For this review, take the finished solid that the model builds, in its own axes (mm). A direction names the side the tool comes from. Coordinates: 2 decimals unless noted, no trailing zeros. Write each loop counter-clockwise with the first axis right and the second up, starting at its lowest first coordinate (ties: lowest second). Pieces come first, ordered by that corner, then holes. Notation, with made-up numbers: (35, 78.5) - (85, 78.5) arc R17 cw to (85, 93.5) - close; hole circle Ø4 at (33, 72). An arc over 180 degrees is marked (long way). Write each question's results on one line, items separated by ' | '.
from build123d import *

# Parameters (mm, degrees)
SKETCH_1_W          = 104
SKETCH_1_H          = 130
EXTRUDE_1_DEPTH     = 70
SHELL_1_T           = -2
SKETCH_4_W          = 21
SKETCH_4_H          = 65
CUT_EXTRUDE_1_DEPTH = 70
SKETCH_6_W          = 16
SKETCH_6_H          = 60
CUT_EXTRUDE_2_DEPTH = 70
SKETCH_13_W         = 3
SKETCH_13_H         = 45
EXTRUDE_5_DEPTH     = 70
FILLET_2_R          = 3


with BuildPart() as part:
    # 草圖1 → 填料-伸長1 (new body)
    with BuildSketch(Plane.XY):
        Rectangle(SKETCH_1_W, SKETCH_1_H)
    extrude(amount=EXTRUDE_1_DEPTH)

    # 薄殼1
    shell_1_openings = [part.faces().sort_by_distance(p)[0] for p in [
        (0, 0, 70),
    ]]
    offset(amount=SHELL_1_T, openings=shell_1_openings, kind=Kind.INTERSECTION)

    # 草圖4 → 除料-伸長1 (cut)
    with BuildSketch(Plane.ZY.offset(52)):
        with Locations((22.5, -28.5)):
            Rectangle(SKETCH_4_W, SKETCH_4_H)
    extrude(amount=-CUT_EXTRUDE_1_DEPTH, mode=Mode.SUBTRACT)

    # 草圖6 → 除料-伸長2 (cut)
    with BuildSketch(Plane(origin=(52, 0, 0), x_dir=(0, 0, -1), z_dir=(1, 0, 0))):
        with Locations((-16.5, 31)):
            Rectangle(SKETCH_6_W, SKETCH_6_H)
    extrude(amount=-CUT_EXTRUDE_2_DEPTH, mode=Mode.SUBTRACT)

    # 草圖13 → 填料-伸長5 (add)
    with BuildSketch(Plane(origin=(52, 0, 0), x_dir=(0, 0, -1), z_dir=(1, 0, 0))):
        with Locations((-31.5, -42.5)):
            Rectangle(SKETCH_13_W, SKETCH_13_H)
    extrude(amount=-EXTRUDE_5_DEPTH)

    # 圓角2
    fillet_2_edges = [part.edges().sort_by_distance(p)[0] for p in [
        (52, -65, 35),
        (-52, -65, 35),
        (-52, 65, 35),
        (52, 65, 35),
    ]]
    fillet(fillet_2_edges, radius=FILLET_2_R)


solid = part.part
Q1. Take a section at C-C on z = 48. State the section outline as (x, y) points.
Results found:
outline: (-52, -62) arc R3 ccw to (-49, -65) - (49, -65) arc R3 ccw to (52, -62) - (52, 62) arc R3 ccw to (49, 65) - (-49, 65) arc R3 ccw to (-52, 62) - close; hole (-50, -63) - (50, -63) - (50, 63) - (-50, 63) - close
Q2. Take a section at A-A on y = -6. State the section outline as (x, z) points.
Results found:
outline: (-52, 0) - (52, 0) - (52, 70) - (50, 70) - (50, 2) - (-50, 2) - (-50, 12) - (-52, 12) - close; (-52, 33) - (-50, 33) - (-50, 70) - (-52, 70) - close
Q3. Take a section at B-B on z = 21.5. State the section outline as (x, y) points.
Results found:
outline: (-52, -62) arc R3 ccw to (-49, -65) - (49, -65) arc R3 ccw to (52, -62) - (52, 1) - (50, 1) - (50, -63) - (-50, -63) - (-50, -61) - (-52, -61) - close; (-52, 4) - (-50, 4) - (-50, 63) - (50, 63) - (50, 61) - (52, 61) - (52, 62) arc R3 ccw to (49, 65) - (-49, 65) arc R3 ccw to (-52, 62) - close
Q4. Wall thickness on line 1 along X through (y, z) = (-7, 43); line 2 along Y through (x, z) = (-13.5, 14.5); line 3 along X through (y, z) = (27, 21): over which ranges is each line inside the solid? List them lowest first. Write a range as from..to.
Results found:
line 1: -52..-50, 50..52 | line 2: -65..-63, 63..65 | line 3: -52..-50
Q5. For faces 1 (the face through (-1, 1, 2)), 2 (the face through (16, -42, 33)), 3 (the face through (16, -20, 32)), list the 3-axis set-ups (+Z, -Z, +X, -X, +Y, -Y) from which the entire face can be reached by the end or side of a thin tool; tool diameter is ignored.
Results found:
face 1: none | face 2: +Z | face 3: +Z, -X
Q6. Mouldability with a two-part tool opening along Y and no side actions: class faces 4 (the face through (-1, 1, 0)), 5 (the face through (-51.1, -64.14, 35.49)), 6 (the face through (50, -1, 36)) as pulls with the +Y half, pulls with the -Y half, needs draft (parallel to the pull), parting line crosses it, or undercut.
Results found:
face 4: needs draft | face 5: pulls with the -Y half | face 6: undercut
Q7. Take a section at D-D on x = -31. State the section outline as (y, z) points.
Results found:
outline: (-65, 0) - (65, 0) - (65, 70) - (63, 70) - (63, 2) - (-63, 2) - (-63, 70) - (-65, 70) - close
Q8. For pin 1 (13 mm diameter, centred on x = 11, y = -48, fed in from +Z); pin 2 (1.6 mm diameter, centred on x = -51, z = 19, fed in from -Y); pin 3 (1 mm diameter, centred on x = 51, z = 20, fed in from -Y), all flat-tipped, find the tip position at first contact; note any pin that passes through.
Results found:
pin 1: z = 33 | pin 2: y = -64.75 | pin 3: y = -64.6
